Check sheet for the drawn part. Datum: minimum x, y, z corner. Units: mm. Round coordinates to 2 decimals unless told otherwise and drop trailing zeros. Loops run counter-clockwise (first coordinate to the right, second up) from the corner with the lowest first, then second, coordinate; pieces in that order, holes last. Notation, with made-up numbers: (78.5, 62) -> (96.5, 62) arc R26 ccw to (96.5, 81) -> close; hole circle Ø10 at (59.25, 33.5). An arc over 180 degrees is marked (long way). Return JSON: item names as keys, results as strings.
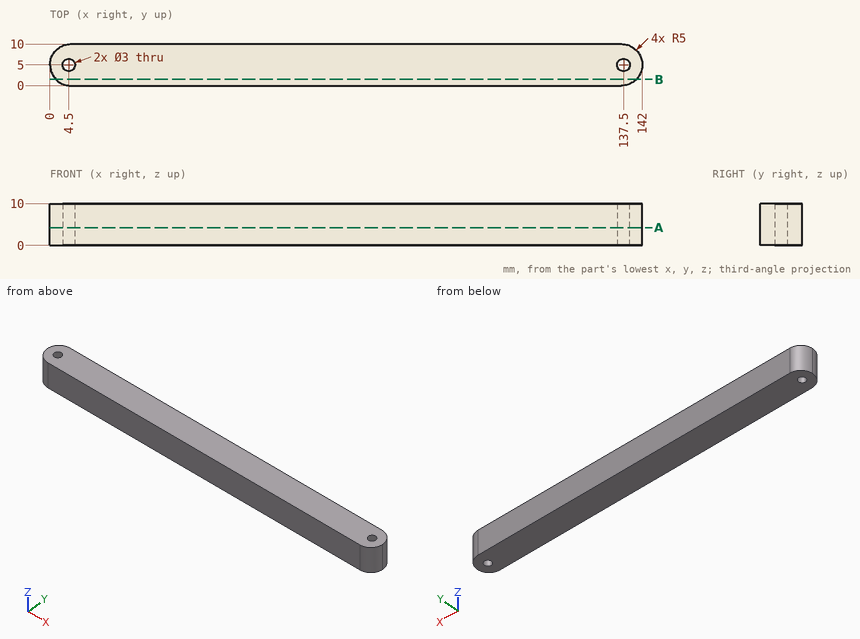
Q1. Section check B-B (y = 1.5). Record the boundary of the cut face in (x, z), then the cut area to 3 significant figures.
Results list:
{"outline": "(1.43, 0) -> (140.57, 0) -> (140.57, 10) -> (1.43, 10) -> close", "area": "1,390 mm^2"}
Q2. Material ranges on line 1 (Y direction, x = 137.5, z = 8.25) (3 decimals); line 2 (X direction, y = 4.5, z = 7.5) (1 decimal); line 3 (X direction, y = 3.75, z = 3), recorded low to high.
Results list:
{"line 1": "0.025 to 3.5, 6.5 to 9.975", "line 2": "0 to 3.1, 5.9 to 136.1, 138.9 to 142", "line 3": "0.16 to 3.67, 5.33 to 136.67, 138.33 to 141.84"}
Q3. Section check A-A (z = 4.25). Count the separate pieces of the cut face and the enclosed holes in it, then the cut area to 3 significant figures.
Results list:
{"separate pieces": "1", "enclosed holes": "2", "area": "1,380 mm^2"}
Q4. Go/stop test with flat-tipped pins: pin 1 (5 mm diameter, centred on x = 68.5, z = 5, fed in from -Y); pin 2 (3 mm diameter, centred on y = 1.5, z = 5, fed in from -X). Record where each tip stops, or that it passes through.
Results list:
{"pin 1": "y = 0", "pin 2": "x = 0.42"}
